Design review of the part shown in the three views and the two pictorial views. Dimensions are in mm from the part's minimum x, y and z. Round coordinates to 2 decimals unless told otherwise and drop trailing zeros. Order: outer loops, then holes, each group sorted by start corner. A loop starts at its lowest first (then second) coordinate and runs counter-clockwise, first axis right, second up.
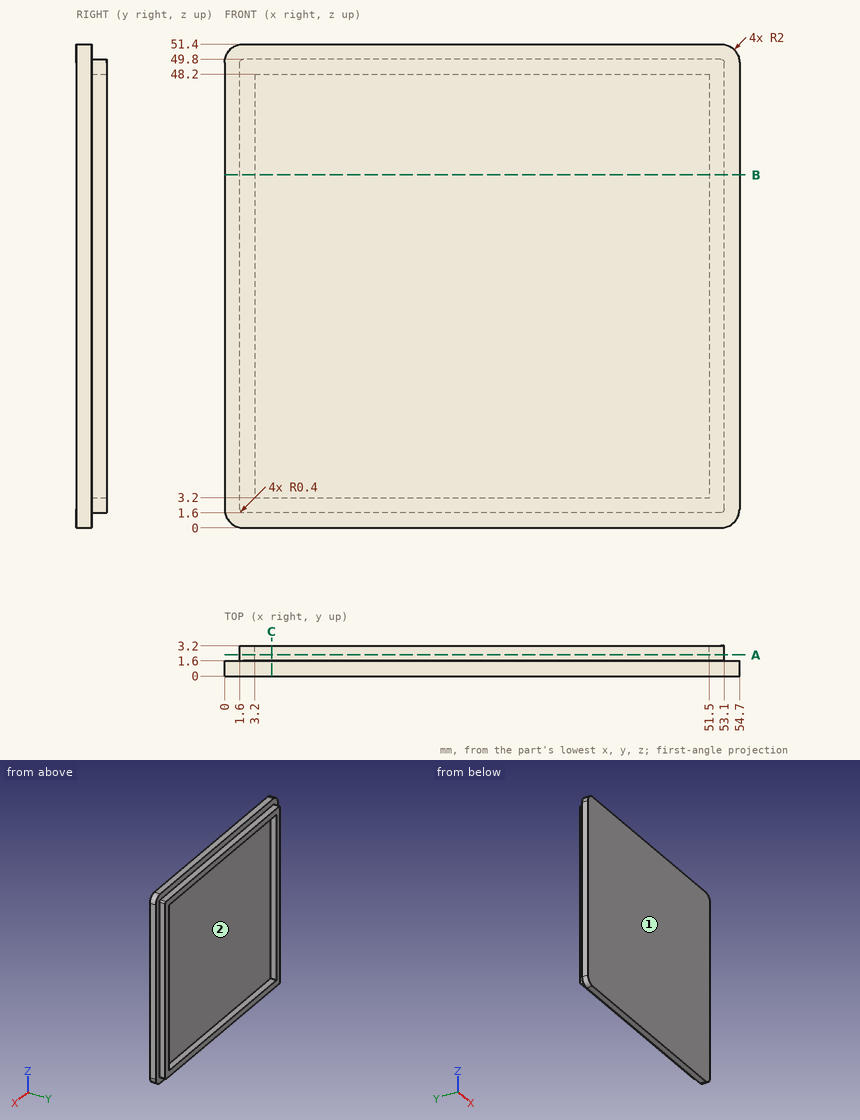
1) Take a section at A-A on y = 2.25. Give the boundary of the cut face in (x, z).
Results:
outline: (1.6, 2) arc R0.4 ccw to (2, 1.6) - (52.7, 1.6) arc R0.4 ccw to (53.1, 2) - (53.1, 49.4) arc R0.4 ccw to (52.7, 49.8) - (2, 49.8) arc R0.4 ccw to (1.6, 49.4) - close; hole (3.2, 3.2) - (51.5, 3.2) - (51.5, 48.2) - (3.2, 48.2) - close
2) To check wall thickness, follow line 1 along Z through (x, y) = (14.5, 2); line 2 along X through (y, z) = (1.85, 17.5); line 3 along Y through (x, z) = (10, 11.5). State the ranges of each line that lie inside material, in increasing order.
Results:
line 1: z = 1.6 to 3.2, 48.2 to 49.8
line 2: x = 1.6 to 3.2, 51.5 to 53.1
line 3: y = 0 to 1.6
3) Take a section at B-B on z = 37.5. Give the boundary of the cut face in (x, y), plus the area to 3 significant figures.
Results:
outline: (0, 0) - (54.7, 0) - (54.7, 1.6) - (53.1, 1.6) - (53.1, 3.2) - (51.5, 3.2) - (51.5, 1.6) - (3.2, 1.6) - (3.2, 3.2) - (1.6, 3.2) - (1.6, 1.6) - (0, 1.6) - close
area: 92.6 mm2
4) The part is to be moulded in two halves that separate along X. For the marked faces 1 and 2, say which applies: released by +X, released by -X, zero draft, split by the parting line, or undercut.
Results:
face 1: zero draft
face 2: undercut
5) Take a section at C-C on x = 5. Give the boundary of the cut face in (y, z).
Results:
outline: (0, 0) - (1.6, 0) - (1.6, 1.6) - (3.2, 1.6) - (3.2, 3.2) - (1.6, 3.2) - (1.6, 48.2) - (3.2, 48.2) - (3.2, 49.8) - (1.6, 49.8) - (1.6, 51.4) - (0, 51.4) - close
6) Clearance check with flat-ended pins moving along their axes: P1, Ø0.8, axis at y = 2.5, z = 20.5, coming from the +X side; P2, Ø10, axis at x = 43.5, z = 25, coming from the +Y side; P3, Ø1.3, axis at x = 32.5, y = 2.5, coming from the +Z side; P4, Ø1.8, axis at x = 23.5, y = 2, coming from the -Z side. State where each tip first meets the part, or that it passes through.
Results:
P1: stops at x = 53.1
P2: stops at y = 1.6
P3: stops at z = 49.8
P4: stops at z = 0
